Here's the drawing with two shaded views (mm, measured from the low corner). I have some questions. A direction names the side the tool comes from. Give positions to 0.01 mm unless a question says otherwise; leave off trailing zeros. Write each loop counter-clockwise with the first axis right and the second up, starting at its lowest first coordinate (ties: lowest second). Pieces come first, ordered by that corner, then holes.
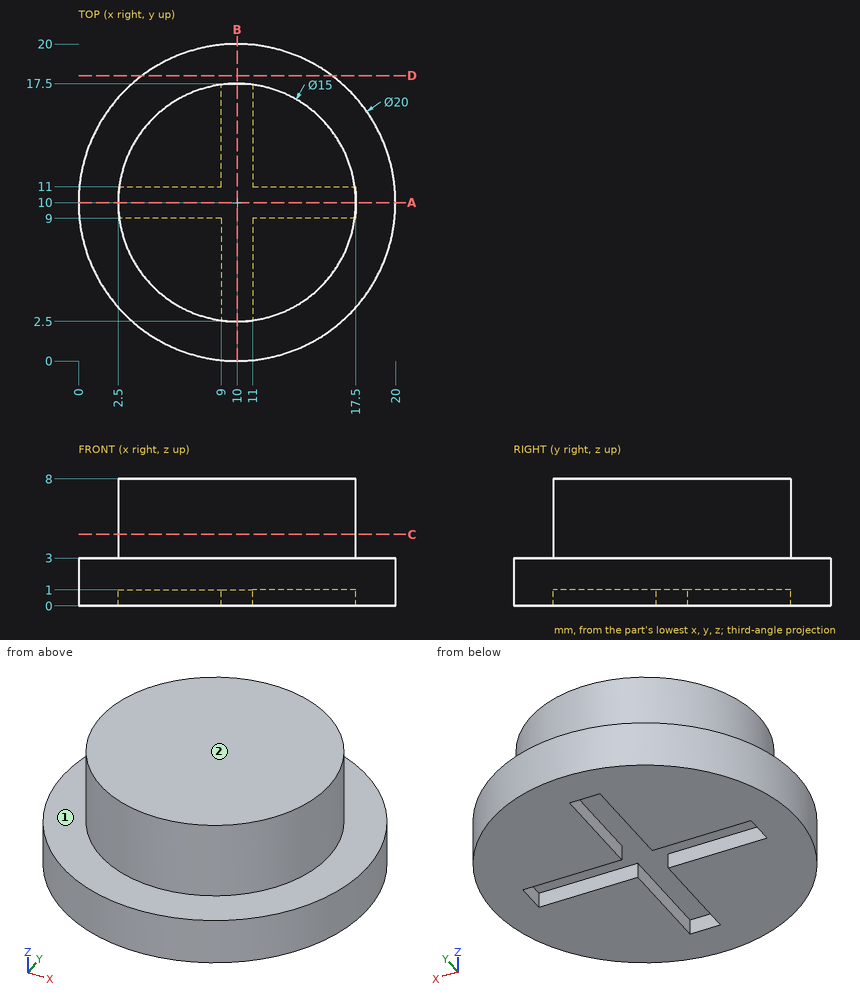
(1) For the marked faces 1 and 2, which set-ups out of +Z, -Z, +X, -X, +Y, -Y let a thin tool reach every point of the face, with its end or its side?
Returned:
face 1: +Z
face 2: +Z, +X, -X, +Y, -Y
(2) Imagine slicing it at C-C, the plane z = 4.5. Write out the boundary of the cut face in (x, y).
Returned:
outline: circle Ø15 at (10, 10)
(3) Will these pins go through, and if not, where does the flat tip stop? P1, Ø0.8, axis at x = 14.5, z = 0.5, coming from the -Y side; P2, Ø3, axis at x = 5, z = 1.5, coming from the -Y side; P3, Ø0.8, axis at x = 6, z = 0.5, coming from the -Y side.
Returned:
P1: stops at y = 0.88
P2: stops at y = 0.63
P3: stops at y = 0.67
(4) Imagine slicing it at A-A, the plane y = 10. Write out the boundary of the cut face in (x, z), plus the area to 3 significant figures.
Returned:
outline: (0, 0) - (2.5, 0) - (2.5, 1) - (17.5, 1) - (17.5, 0) - (20, 0) - (20, 3) - (17.5, 3) - (17.5, 8) - (2.5, 8) - (2.5, 3) - (0, 3) - close
area: 120 mm2
(5) Imagine slicing it at D-D, the plane y = 18. Write out the boundary of the cut face in (x, z), plus the area to 3 significant figures.
Returned:
outline: (4, 0) - (16, 0) - (16, 3) - (4, 3) - close
area: 36.0 mm2
(6) If I drill on L1, parallel to Z at x = 19, y = 10.5; L2, parallel to X at y = 3, z = 0.75; L3, parallel to Z at x = 9.5, y = 4.25, over which ranges is the centre line in solid material (lowest first)?
Returned:
L1: z = 0 to 3
L2: x = 2.86 to 9, 11 to 17.14
L3: z = 1 to 8
